```python
from build123d import *

# Parameters (mm, degrees)
SKETCH1_W           = 64
SKETCH1_H           = 79
BOSS_EXTRUDE1_DEPTH = 2
SKETCH2_W           = 64
SKETCH2_H           = 79
BOSS_EXTRUDE6_DEPTH = 4
FILLET1_R           = 2
FILLET2_R           = 2
FILLET3_R           = 2
FILLET4_R           = 2
SKETCH4_R           = 2
CUT_EXTRUDE1_DEPTH  = 2
SKETCH6_R           = 1.25
CUT_EXTRUDE2_DEPTH  = 4
FILLET5_R           = 1


with BuildPart() as part:
    # Sketch1 → Boss-Extrude1 (new body)
    with BuildSketch(Plane.XY):
        Rectangle(SKETCH1_W, SKETCH1_H)
    extrude(amount=BOSS_EXTRUDE1_DEPTH)

    # Sketch2 → Boss-Extrude6 (add)
    with BuildSketch(Plane.XY.offset(2)):
        Rectangle(SKETCH2_W, SKETCH2_H)
        Polygon((-30, 31.5), (-24, 37.5), (24, 37.5), (30, 31.5), (30, -31.5), (24, -37.5), (-24, -37.5), (-30, -31.5), align=None, mode=Mode.SUBTRACT)
    extrude(amount=BOSS_EXTRUDE6_DEPTH)

    # Fillet1
    fillet1_edges = [part.edges().sort_by_distance(p)[0] for p in [
        (-32, -39.5, 3),
    ]]
    fillet(fillet1_edges, radius=FILLET1_R)

    # Fillet2
    fillet2_edges = [part.edges().sort_by_distance(p)[0] for p in [
        (32, -39.5, 3),
    ]]
    fillet(fillet2_edges, radius=FILLET2_R)

    # Fillet3
    fillet3_edges = [part.edges().sort_by_distance(p)[0] for p in [
        (32, 39.5, 3),
    ]]
    fillet(fillet3_edges, radius=FILLET3_R)

    # Fillet4
    fillet4_edges = [part.edges().sort_by_distance(p)[0] for p in [
        (-32, 39.5, 3),
    ]]
    fillet(fillet4_edges, radius=FILLET4_R)

    # Sketch4 → Cut-Extrude1 (cut)
    with BuildSketch(Plane(origin=(0, 0, 0), x_dir=(-1, 0, 0), z_dir=(0, 0, -1))):
        with Locations((29, 36.5)):
            Circle(SKETCH4_R)
        with Locations((29, -36.5)):
            Circle(SKETCH4_R)
        with Locations((-29, -36.5)):
            Circle(SKETCH4_R)
        with Locations((-29, 36.5)):
            Circle(SKETCH4_R)
    extrude(amount=-CUT_EXTRUDE1_DEPTH, mode=Mode.SUBTRACT)

    # Sketch6 → Cut-Extrude2 (cut)
    with BuildSketch(Plane(origin=(0, 0, 2), x_dir=(-1, 0, 0), z_dir=(0, 0, -1))):
        with Locations((29, 36.5)):
            Circle(SKETCH6_R)
        with Locations((29, -36.5)):
            Circle(SKETCH6_R)
        with Locations((-29, -36.5)):
            Circle(SKETCH6_R)
        with Locations((-29, 36.5)):
            Circle(SKETCH6_R)
    extrude(amount=-CUT_EXTRUDE2_DEPTH, mode=Mode.SUBTRACT)

    # Fillet5
    fillet5_edges = [part.edges().sort_by_distance(p)[0] for p in [
        (0, -39.5, 0),
        (-31.414213562, -38.914213562, 0),
        (32, 0, 0),
        (31.414213562, -38.914213562, 0),
        (0, 39.5, 0),
        (31.414213562, 38.914213562, 0),
        (-32, 0, 0),
        (-31.414213562, 38.914213562, 0),
    ]]
    fillet(fillet5_edges, radius=FILLET5_R - 0.0001)  # a hair under: the kernel refuses the full size


solid = part.part
```
Source: CAD feature listing. Evaluate the final solid. Frame: model axes, mm. A direction names the side the tool comes from. Round coordinates to 2 decimals unless told otherwise and drop trailing zeros. Order: outer loops, then holes, each group sorted by start corner. A loop starts at its lowest first (then second) coordinate and runs counter-clockwise, first axis right, second up. Notation, with made-up numbers: (-32.5, 51) -> (-21.5, 51) arc R22 ccw to (-21.5, 64) -> close; hole circle Ø10 at (53, 61). An arc over 180 degrees is marked (long way). Use CSV: the item, a comma, the result in double quotes.
(1) Section C-C on z = 3.3. Return the cut outline in (x, y), and give its area (3 significant figures).
Report:
outline,"(-32, -37.5) arc R2 ccw to (-30, -39.5) -> (30, -39.5) arc R2 ccw to (32, -37.5) -> (32, 37.5) arc R2 ccw to (30, 39.5) -> (-30, 39.5) arc R2 ccw to (-32, 37.5) -> close; hole circle Ø2.5 at (-29, -36.5); hole circle Ø2.5 at (-29, 36.5); hole (-30, -31.5) -> (-24, -37.5) -> (24, -37.5) -> (30, -31.5) -> (30, 31.5) -> (24, 37.5) -> (-24, 37.5) -> (-30, 31.5) -> close; hole circle Ø2.5 at (29, -36.5); hole circle Ø2.5 at (29, 36.5)"
area,"605 mm^2"
(2) First-contact query: pin 1 Ø1.5 at (x, y) = (29, -36.5) entering from -Z; pin 2 Ø2 at (x, y) = (29.5, -36) entering from -Z. Flat tips, straight axial feed; report the tip coordinate or a pass-through.
Report:
pin 1,"through"
pin 2,"z = 2"
(3) Section D-D on x = 2. Return the cut outline in (y, z).
Report:
outline,"(-39.5, 1) arc R1 ccw to (-38.5, 0) -> (38.5, 0) arc R1 ccw to (39.5, 1) -> (39.5, 6) -> (37.5, 6) -> (37.5, 2) -> (-37.5, 2) -> (-37.5, 6) -> (-39.5, 6) -> close"
(4) Pull-direction query (X, two-part tool) for faces 4 (the face through (28.077, -38.274, 0.986)), 5 (the face through (31.43, 38.9, 3.46)), 6 (the face through (0, 1, 0)), 7 (the face through (27, 34.5, 4)); classes: +X half, -X half, draft (parallel to the pull), parting line (faces both ways), or undercut.
Report:
face 4,"undercut"
face 5,"+X half"
face 6,"draft"
face 7,"undercut"
(5) Access query for faces 1 (the face through (30, 0, 4)), 2 (the face through (27.845, -36.979, 3.972)), 3 (the face through (-29.923, -38.274, 0.986)). Directions: +Z, -Z, +X, -X, +Y, -Y. A direction counts if a zero-diameter tool reaches every point of the face in a straight line with its end or side. Return the directions, or none.
Report:
face 1,"+Z"
face 2,"+Z, -Z"
face 3,"-Z"
(6) Section A-A on y = 36.5. Count the separate pieces of the cut face and the enclosed holes in it, and give its area (3 significant figures).
Report:
separate pieces,"3"
enclosed holes,"0"
area,"148 mm^2"
(7) Ray query, L1, parallel to Y at x = 29, z = 1.25; L2, parallel to X at y = 17, z = 3; L3, parallel to Y at x = 29, z = 5.2. Return the intervals inside material, ascending.
Report:
L1,"-39.5 to -38.5, -34.5 to 34.5, 38.5 to 39.5"
L2,"-32 to -30, 30 to 32"
L3,"-39.5 to -37.75, -35.25 to -32.5, 32.5 to 35.25, 37.75 to 39.5"
